Could you check a few things on this model? Use its own coordinates, in mm. Give positions to 0.01 mm unless a question says otherwise; leave off trailing zeros. Loops run counter-clockwise (first coordinate to the right, second up) from the corner with the lowest first, then second, coordinate; pieces in that order, holes last. Notation, with made-up numbers: (2, 58.5) -> (19, 58.5) arc R27 cw to (19, 95.5) -> close; hole circle Ø2 at (10.25, 21.5). An arc over 180 degrees is marked (long way). Write each question's results on one line, items separated by ' | '. Start each with the question number.
Q1. If I drill on line 1 along X through (y, z) = (-27, 82.5); line 2 along Y through (x, z) = (8.5, 58); line 3 along X through (y, z) = (-12.5, 129), over which ranges is the centre line in solid material (lowest first)?
Q2. If we section it at B-B, the plane z = 226: List the corners of the cut face in (x, y) for me, plus the area to 3 significant figures.
Q3. Will these pins go through, and if not, where does the flat tip stop? P1, Ø3, axis at x = 15, z = 105, coming from the +Y side; P2, Ø2, axis at y = -15.5, z = 27, coming from the -X side; P3, Ø5, axis at x = -8.5, z = 196, coming from the +Y side.
Q4. If we section it at A-A, the plane z = 64: List the corners of the cut face in (x, y) for me, plus the area to 3 significant figures.
from build123d import *

# Parameters (mm, degrees)
F0_R      = 30.5
F2_DEPTH  = 111
F2_FACE_R = 30.5
F3_R      = 18.5
F5_R      = 5
F6_R      = 5
F4_FACE_R = 18.5
F8_R      = 13.3


with BuildPart() as f2:
    # F0 (on Top) → F2 (new body)
    with BuildSketch(Plane.XY):
        Circle(F0_R)
    extrude(amount=F2_DEPTH)

    # F2_face (on face) → F4 section 0
    with BuildSketch(Plane.XY.offset(111)):
        Circle(F2_FACE_R)
    # F3 (on offset) → F4 section 1
    with BuildSketch(Plane.XY.offset(152.5)):
        Circle(F3_R)
    loft()

    # F5
    f5_edges = [f2.edges().sort_by_distance(p)[0] for p in [
        (-30.5, 0, 111),
    ]]
    fillet(f5_edges, radius=F5_R)

    # F6
    f6_edges = [f2.edges().sort_by_distance(p)[0] for p in [
        (-30.5, 0, 0),
    ]]
    fillet(f6_edges, radius=F6_R)

    # F4_face (on face) → F9 section 0
    with BuildSketch(Plane.XY.offset(152.5)):
        Circle(F4_FACE_R)
    # F8 (on offset) → F9 section 1
    with BuildSketch(Plane.XY.offset(240.5)):
        Circle(F8_R)
    loft()


solid = f2.part
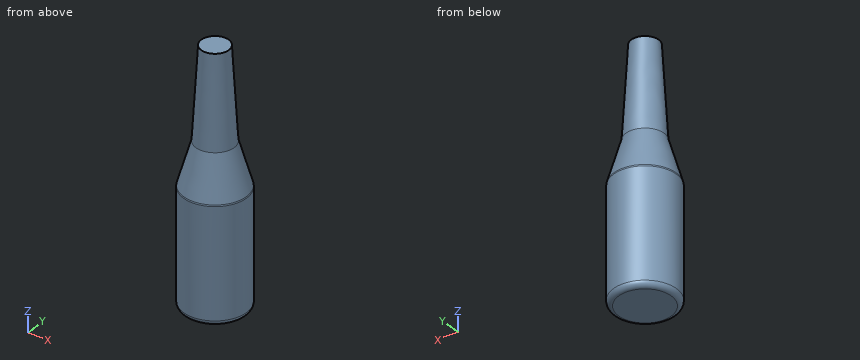
Final values:
1) line 1: x = -14.19 to 14.19 | line 2: y = -29.29 to 29.29 | line 3: x = -21.99 to 21.99
2) outline: circle Ø28.31 at (0, 0) | area: 630 mm²
3) P1: stops at y = 27.35 | P2: stops at x = -26.83 | P3: stops at y = 14.77
4) outline: circle Ø61 at (0, 0) | area: 2,920 mm²
